Model file for the job. Use its own axes, mm. Face numbers are marked on the shaded views. A direction names the side the tool comes from. Coordinates: 2 decimals unless noted, no trailing zeros. Order: outer loops, then holes, each group sorted by start corner. A loop starts at its lowest first (then second) coordinate and runs counter-clockwise, first axis right, second up.
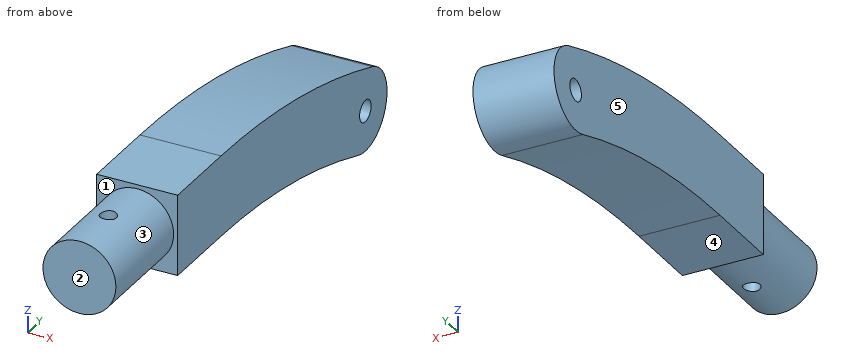
from build123d import *

# Parameters (mm, degrees)
SKETCH2_W           = 30
SKETCH2_H           = 30
SKETCH3_R           = 13.5
BOSS_EXTRUDE1_DEPTH = 40
BOSS_EXTRUDE2_DEPTH = 30
CUT_EXTRUDE1_REACH  = 153.523
SKETCH5_R           = 4
CUT_EXTRUDE2_REACH  = 155.212
SKETCH6_R           = 3


with BuildPart() as part:
    # Sweep1: sweep along a path in Sketch1
    with BuildLine(Plane(origin=(0, 0, 0), x_dir=(0, 0, -1), z_dir=(1, 0, 0))) as sweep1_path:
        Line((0, 0), (0, 30))
        ThreePointArc((0, 30), (4.320432104, 80.730593618), (17.157287525, 130))
    # Sketch2 → Sweep1 (sweep)
    with BuildSketch(Plane(origin=(0, 0, 0), x_dir=(1, 0, 0), z_dir=(0, 1, 0))):
        Rectangle(SKETCH2_W, SKETCH2_H)
    sweep(path=sweep1_path.line)

    # Sketch3 → Boss-Extrude1 (add)
    with BuildSketch(Plane.XZ):
        with Locations(Location((0, 0, 0), (0, 0, 270))):
            Circle(SKETCH3_R)
    extrude(amount=BOSS_EXTRUDE1_DEPTH)

    # Sketch4 → Boss-Extrude2 (add)
    with BuildSketch(Plane(origin=(15, 0, 0), x_dir=(0, 0, -1), z_dir=(1, 0, 0))):
        with BuildLine():
            Line((3.015151902, 135), (31.299423149, 125))
            ThreePointArc((31.299423149, 125), (22.157287525, 144.142135624), (3.015151902, 135))
        make_face()
    extrude(amount=-BOSS_EXTRUDE2_DEPTH)

    # Sketch5 → Cut-Extrude1 (cut, up to next)
    with BuildSketch(Plane(origin=(15, 0, 0), x_dir=(0, 0, -1), z_dir=(1, 0, 0)), mode=Mode.PRIVATE) as cut_extrude1_sk1:
        with Locations((17.157287525, 130)):
            Circle(SKETCH5_R)
    cut_extrude1_tool1 = extrude(cut_extrude1_sk1.sketch, amount=-CUT_EXTRUDE1_REACH, mode=Mode.PRIVATE) & part.part
    add(cut_extrude1_tool1.solids().sort_by_distance((15, 130, -17.157288))[0], mode=Mode.SUBTRACT)

    # Sketch6 → Cut-Extrude2 (cut, up to next)
    with BuildSketch(Plane.XY.offset(15), mode=Mode.PRIVATE) as cut_extrude2_sk1:
        with Locations((0, -20)):
            Circle(SKETCH6_R)
    cut_extrude2_tool1 = extrude(cut_extrude2_sk1.sketch, amount=-CUT_EXTRUDE2_REACH, mode=Mode.PRIVATE) & part.part
    add(cut_extrude2_tool1.solids().sort_by_distance((0, -20, 15))[0], mode=Mode.SUBTRACT)


solid = part.part
Q1. Cut at B-B, the plane z = -17.5. List the corners of the cut face in (x, y), plus the area to 3 significant figures.
Established:
outline: (-15, 67.67) - (15, 67.67) - (15, 126.01) - (-15, 126.01) - close; (-15, 133.99) - (15, 133.99) - (15, 145) - (-15, 145) - close
area: 2,080 mm2
Q2. Which spindle directions (+Z, -Z, +X, -X, +Y, -Y) get a long thin tool onto all of the face, cutting with end or side? Do the marked faces 1 and 2. Say none if no direction does.
Established:
face 1: -Y
face 2: +Z, -Z, +X, -X, -Y
Q3. Mould opens along X. For the marked faces 3, 4 and 5 say: pulls with the +X half, pulls with the -X half, needs draft (parallel to the pull), parting line crosses it, or undercut.
Established:
face 3: parting line crosses it
face 4: needs draft
face 5: pulls with the -X half
Q4. Cut at A-A, the plane x = 0. List the corners of the cut face in (y, z), plus the area to 3 significant figures.
Established:
outline: (-40, -13.5) - (-23, -13.5) - (-23, 13.5) - (-40, 13.5) - close; (-17, -13.5) - (0, -13.5) - (0, -15) - (30, -15) arc R285 cw to (125, -31.3) arc R15 ccw to (135, -3.02) arc R315 ccw to (30, 15) - (0, 15) - (0, 13.5) - (-17, 13.5) - close; hole circle Ø8 at (130, -17.16)
area: 5,180 mm2
Q5. Drop flat-ended pins along their axis: P1, Ø5, axis at x = 2.5, z = -16, coming from the +Y side; P2, Ø1, axis at x = 1.5, y = -4, coming from the +Z side; P3, Ø8, axis at x = 0.5, y = 65, coming from the -Z side; P4, Ø9, axis at x = 0, y = 11, coming from the -Z side. Give the stop position or say it passes through.
Established:
P1: stops at y = 145
P2: stops at z = 13.46
P3: stops at z = -17.68
P4: stops at z = -15
Q6. Probe line 1 (X direction, y = -20, z = 0.5); line 2 (Z direction, x = -0.75, y = -32.5); line 3 (Z direction, x = 11, y = 29.5). List the from-to ranges inside material, lowest first.
Established:
line 1: x = -13.49 to -3, 3 to 13.49
line 2: z = -13.48 to 13.48
line 3: z = -15 to 15
Q7. Cut at D-D, the plane z = 0. List the corners of the cut face in (x, y).
Established:
outline: (-15, 0) - (-13.5, 0) - (-13.5, -40) - (13.5, -40) - (13.5, 0) - (15, 0) - (15, 126.05) - (-15, 126.05) - close; hole circle Ø6 at (0, -20)
Q8. Cut at C-C, the plane y = 130. List the corners of the cut face in (x, z).
Established:
outline: (-15, -32.16) - (15, -32.16) - (15, -21.16) - (-15, -21.16) - close; (-15, -13.16) - (15, -13.16) - (15, -1.29) - (-15, -1.29) - close
